from build123d import *

# Parameters (mm, degrees)
SALIENTE_EXTRUIR1_DEPTH = 35


with BuildPart() as part:
    # Croquis3 → Saliente-Extruir1 (new body)
    with BuildSketch(Plane(origin=(0, 0, 0), x_dir=(0, 0, -1), z_dir=(1, 0, 0))):
        Polygon((-73.800980209, -80.62474503), (-123.800980209, -80.62474503), (-73.800980209, 251.36525497), (-23.800980209, 251.36525497), align=None)
        Polygon((-48.800980209, 85.37025497), (-54.775537144, 45.700391836), (-11.85186634, 45.700391836), (-23.800980209, 85.37025497), align=None)
        Polygon((-23.800980209, 85.37025497), (-11.85186634, 45.700391836), (26.199019791, -80.62474503), (76.199019791, -80.62474503), (-23.800980209, 251.36525497), (-40.467646876, 140.701921636), align=None)
    extrude(amount=SALIENTE_EXTRUIR1_DEPTH)


solid = part.part
Design review of the part built by this model. Coordinates are the model's own, in mm. A direction names the side the tool comes from. Give positions to 0.01 mm unless a question says otherwise; leave off trailing zeros. Order: outer loops, then holes, each group sorted by start corner. A loop starts at its lowest first (then second) coordinate and runs counter-clockwise, first axis right, second up.
1. Add section D-D, the plane y = 68. State the section outline as (x, z) points, then the cut area to 3 significant figures.
Solution:
outline: (0, -31.43) - (35, -31.43) - (35, 101.42) - (0, 101.42) - close
area: 4,650 mm2
2. Mouldability with a two-part tool opening along Z and no side actions: class faces 4 (the flat face through (17.255, -16.578, 64.155)), 5 (the flat face through (17.255, -16.578, -6.907)), 6 (the flat face through (17, -80.625, 98)), 7 (the flat face through (17.26, 83.05, -26.9)) as +Z half, -Z half, draft (parallel to the pull), parting line (faces both ways), or undercut.
Solution:
face 4: undercut
face 5: undercut
face 6: draft
face 7: -Z half
3. Add section C-C, the plane z = 28. State the section outline as (x, y) points, then the cut area to 3 significant figures.
Solution:
outline: (0, 45.7) - (35, 45.7) - (35, 85.37) - (0, 85.37) - close; (0, 99.31) - (35, 99.31) - (35, 251.37) - (0, 251.37) - close
area: 6,710 mm2
4. Tool access review of faces 1 (the flat face through (17.26, 83.05, 99.15)), 2 (the flat face through (17, 45.7, 34)), 3 (the flat face through (17.26, 113.42, 32.25)): name each direction out of +Z, -Z, +X, -X, +Y, -Y from which nothing blocks a thin tool from reaching the whole face with its end or side.
Solution:
face 1: +Z, +X, -X, +Y
face 2: +X, -X, -Y
face 3: +X, -X
5. Add section A-A, the plane y = -5. State the section outline as (x, z) points, then the cut area to 3 significant figures.
Solution:
outline: (0, -53.42) - (35, -53.42) - (35, -3.42) - (0, -3.42) - close; (0, 62.41) - (35, 62.41) - (35, 112.41) - (0, 112.41) - close
area: 3,500 mm2
6. To check wall thickness, follow L1, parallel to Z at x = 6, y = -64.5; L2, parallel to Z at x = 30, y = 116; L3, parallel to Z at x = 14.5, y = 231. State the ranges of each line that lie inside material, in increasing order.
Solution:
L1: z = -71.34 to -21.34, 71.37 to 121.37
L2: z = -16.97 to 33.03, 44.19 to 94.19
L3: z = 17.67 to 76.87
7. Add section B-B, the plane x = 13.5. State the section outline as (y, z) points.
Solution:
outline: (-80.62, -76.2) - (251.37, 23.8) - (251.37, 73.8) - (-80.62, 123.8) - (-80.62, 73.8) - (45.7, 54.78) - (45.7, 11.85) - (-80.62, -26.2) - close; hole (85.37, 23.8) - (140.7, 40.47) - (85.37, 48.8) - close
8. For pin 1 Ø1.5 at (x, y) = (5.5, 148) entering from -Z; pin 2 Ø10.5 at (x, z) = (17, 31) entering from -Y; pin 3 Ø3 at (x, y) = (16.5, 51) entering from -Z, all flat-tipped, find the tip position at first contact; note any pin that passes through.
Solution:
pin 1: stops at z = -7.56
pin 2: stops at y = 45.7
pin 3: stops at z = -37
